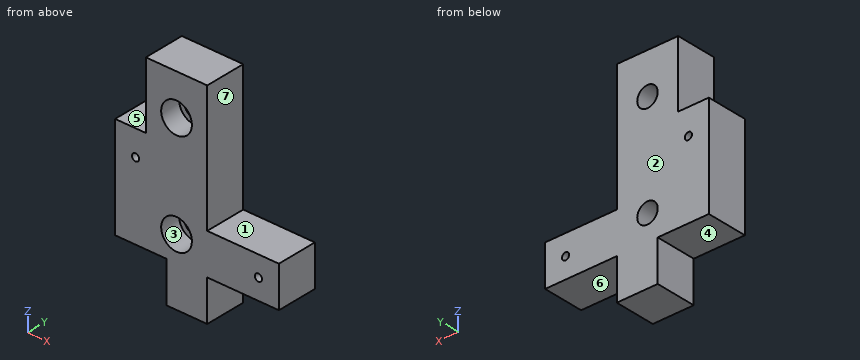
from build123d import *

# Parameters (mm, degrees)
SKETCH_1_W          = 16
SKETCH_1_H          = 23
SKETCH_1_R          = 0.35
EXTRUDE_1_DEPTH     = 4
SKETCH_2_R          = 1
CUT_EXTRUDE_1_DEPTH = 29.301943396
SKETCH_3_R          = 1.5
CUT_EXTRUDE_2_DEPTH = 2
SKETCH_4_W          = 6
SKETCH_4_H          = 2.5
SKETCH_4_W_2        = 7
SKETCH_4_H_2        = 4
SKETCH_4_W_3        = 5
CUT_EXTRUDE_3_DEPTH = 29.301943396


with BuildPart() as part:
    # 草图1 → 凸台-拉伸1 (new body)
    with BuildSketch(Plane(origin=(0, 0, 0), x_dir=(1, 0, 0), z_dir=(0, 1, 0))):
        with Locations((8, -11.5)):
            Rectangle(SKETCH_1_W, SKETCH_1_H)
        with Locations(Location((14, -6, 0), (0, 0, 270))):
            Circle(SKETCH_1_R, mode=Mode.SUBTRACT)
        with Locations(Location((2, -11.5, 0), (0, 0, 270))):
            Circle(SKETCH_1_R, mode=Mode.SUBTRACT)
    extrude(amount=EXTRUDE_1_DEPTH)

    # 草图2 → 切除-拉伸1 (cut, through all)
    with BuildSketch(Plane.XZ):
        with Locations(Location((6, 16.5, 0), (0, 0, 270))):
            Circle(SKETCH_2_R)
        with Locations(Location((6, 6.5, 0), (0, 0, 270))):
            Circle(SKETCH_2_R)
    extrude(amount=-CUT_EXTRUDE_1_DEPTH, mode=Mode.SUBTRACT)

    # 草图3 → 切除-拉伸2 (cut)
    with BuildSketch(Plane.XZ):
        with Locations(Location((6, 16.5, 0), (0, 0, 270))):
            Circle(SKETCH_3_R)
        with Locations(Location((6, 6.5, 0), (0, 0, 270))):
            Circle(SKETCH_3_R)
    extrude(amount=-CUT_EXTRUDE_2_DEPTH, mode=Mode.SUBTRACT)

    # 草图4 → 切除-拉伸3 (cut, through all)
    with BuildSketch(Plane.XZ):
        with Locations((6, 21.75)):
            Rectangle(SKETCH_4_W, SKETCH_4_H)
        Polygon((3, 23), (0, 23), (0, 14), (3, 14), (3, 20.5), align=None)
        Polygon((16, 23), (9, 23), (9, 20.5), (9, 8), (16, 8), align=None)
        with Locations((12.5, 2)):
            Rectangle(SKETCH_4_W_2, SKETCH_4_H_2)
        with Locations((2.5, 2)):
            Rectangle(SKETCH_4_W_3, SKETCH_4_H_2)
    extrude(amount=-CUT_EXTRUDE_3_DEPTH, mode=Mode.SUBTRACT)


solid = part.part
CAD build for the part. Positions are in the model's coordinates, mm. Face numbers are marked on the shaded views. A direction names the side the tool comes from. Give positions to 0.01 mm unless a question says otherwise; leave off trailing zeros. Loops run counter-clockwise (first coordinate to the right, second up) from the corner with the lowest first, then second, coordinate; pieces in that order, holes last. Notation, with made-up numbers: M 33,-8 L 46,-8 A13 cw 46,-1 Z; hole C -32.75,35.25 d6. An arc over 180 degrees is marked long. Answer in a Markdown table with one row per item. Add a question column.
Item 1: Band-saw the part on A-A on z = 16.5. Give the cut face in (x, y), then the cut area to 3 significant figures.
Item 2: Band-saw the part on C-C on y = 1.4. Give the cut face in (x, z), then the cut area to 3 significant figures.
Item 3: Band-saw the part on D-D on z = 6. Give the cut face in (x, y).
Item 4: Mould opens along Z. For the marked faces 1, 2, 3 and 4 say: +Z half, -Z half, draft (parallel to the pull), parting line (faces both ways), or undercut.
Item 5: Drop flat-ended pins along their axis: P1, Ø0.9, axis at x = 1.5, y = 3, coming from the +Z side; P2, Ø2, axis at y = 2, z = 2, coming from the +X side; P3, Ø2.5, axis at x = 6, z = 16.5, coming from the -Y side. Give the stop position or say it passes through.
Item 6: Band-saw the part on B-B on x = 2. Give the cut face in (y, z).
Item 7: Tool access for the marked faces 5, 6 and 7: list every direction of +Z, -Z, +X, -X, +Y, -Y with a clear straight run to the whole face (end or side of a thin tool).
Item 8: Probe probe 1 along X at (y, z) = (0.65, 6.5); probe 2 along Z at (x, y) = (6.75, 0.7); probe 3 along X at (y, z) = (2.6, 6.5). List the from-to ranges inside material, lowest first.
Reply:
| question | item | result |
|---|---|---|
| 1 | outline | M 3,0 L 4.5,0 L 4.5,2 L 5,2 L 5,4 L 3,4 Z; M 7,2 L 7.5,2 L 7.5,0 L 9,0 L 9,4 L 7,4 Z |
| 1 | area | 14.0 mm^2 |
| 2 | outline | M 0,4 L 5,4 L 5,0 L 9,0 L 9,4 L 16,4 L 16,8 L 9,8 L 9,20.5 L 3,20.5 L 3,14 L 0,14 Z; hole C 2,11.5 d0.7; hole C 6,6.5 d3; hole C 6,16.5 d3; hole C 14,6 d0.7 |
| 2 | area | 158 mm^2 |
| 3 | outline | M 0,0 L 4.59,0 L 4.59,2 L 5.13,2 L 5.13,4 L 0,4 Z; M 6.87,2 L 7.41,2 L 7.41,0 L 13.65,0 L 13.65,4 L 6.87,4 Z; M 14.35,0 L 16,0 L 16,4 L 14.35,4 Z |
| 4 | face 1 | +Z half |
| 4 | face 2 | draft |
| 4 | face 3 | undercut |
| 4 | face 4 | -Z half |
| 5 | P1 | stops at z = 14 |
| 5 | P2 | stops at x = 9 |
| 5 | P3 | stops at y = 2 |
| 6 | outline | M 0,4 L 4,4 L 4,11.15 L 0,11.15 Z; M 0,11.85 L 4,11.85 L 4,14 L 0,14 Z |
| 7 | face 5 | +Z, -X, +Y, -Y |
| 7 | face 6 | -Z, +X, +Y, -Y |
| 7 | face 7 | +Z, +X, +Y, -Y |
| 8 | probe 1 | x = 0 to 4.5, 7.5 to 16 |
| 8 | probe 2 | z = 0 to 5.2, 7.8 to 15.2, 17.8 to 20.5 |
| 8 | probe 3 | x = 0 to 5, 7 to 16 |
